Geometry: final body of the model. Coordinates: model frame, mm. Give positions to 0.01 mm unless a question says otherwise; leave off trailing zeros. Write each loop counter-clockwise with the first axis right and the second up, starting at its lowest first coordinate (ties: lowest second). Pieces come first, ordered by that corner, then holes.
Autodesk Inventor part; units mm, degrees
ref_plane "YZ Plane" through (0, 0, 0) normal (1, 0, 0) x (0, 1, 0)
ref_plane "XZ Plane" through (0, 0, 0) normal (0, 1, 0) x (-1, 0, 0)
ref_plane "XY Plane" through (0, 0, 0) normal (0, 0, 1) x (1, 0, 0)
sketch "Sketch3" plane through (0, 0, 0) normal (0, 1, 0) x (-1, 0, 0)
  line L0 (-56.572, -4.0671) -> (-56.572, -54.0671)
  line L1 (-6.572, -54.0671) -> (-6.572, -4.0671)
  line L2 (-6.572, -4.0671) -> (-35.572, -4.0671)
  line L3 (-35.572, -4.0671) -> (-35.572, -8.0671)
  line L4 (-35.572, -8.0671) -> (-27.572, -8.0671)
  line L5 (-27.572, -8.0671) -> (-27.572, -4.0671)
  line L6 (-27.572, -4.0671) -> (-56.572, -4.0671)
  line L7 (-6.572, -29.0671) -> (-22.7851, -29.0671) construction
  line L8 (-6.572, -54.0671) -> (-35.572, -54.0671)
  line L9 (-35.572, -54.0671) -> (-35.572, -50.0671)
  line L10 (-35.572, -50.0671) -> (-27.572, -50.0671)
  line L11 (-27.572, -50.0671) -> (-27.572, -54.0671)
  line L12 (-27.572, -54.0671) -> (-56.572, -54.0671)
  line L13 (-21.572, -4.0671) -> (-21.572, -19.0671) construction
  line L14 (-21.572, -19.0671) -> (-6.572, -19.0671) construction
  line L15 (-56.572, -19.0671) -> (-41.572, -19.0671) construction
  line L16 (-56.572, -39.0671) -> (-41.572, -39.0671) construction
  line L17 (-21.572, -54.0671) -> (-21.572, -39.0671) construction
  line L18 (-21.572, -39.0671) -> (-6.572, -39.0671) construction
  circle A0 centre (-21.572, -19.0671) radius 3
  circle A1 centre (-41.572, -19.0671) radius 3
  circle A2 centre (-41.572, -39.0671) radius 3
  circle A3 centre (-21.572, -39.0671) radius 3
  point P0 (-35.572, -4.0671)
  dimension "d36" = 50
  dimension "d37" = 50
  dimension "d38" = 4
  dimension "d40" = 15
  dimension "d41" = 6
  dimension "d46" = 8
extrude "Extrusion3" add sketch "Sketch3" along normal blind 600 contours L6 L3 L4 L5 L2 L1 L8 L11 L10 L9 L12 L0 | A0 | A1 | A2 | A3
extrude "Extrusion6" cut sketch "Sketch3" along normal blind 30 contours A0 | A1 | A2 | A3
extrude "Extrusion7" cut sketch "Sketch3" against normal blind 30 from surface at 600 contours A0 | A1 | A2 | A3
equation "\"d36\" = inner_leg_width"
equation "\"d37\" = inner_leg_width"
equation "\"d38\" = cabel_shaft_size"
equation "\"d40\" = edge_to_hole"
equation "\"d41\" = hole_diameter"
equation "\"d46\" = 2 * cabel_shaft_size"
equation "\"d12\" = height"
equation "\"d42\" = hole_depth"
equation "\"d44\" = hole_depth"
equation "\"cabel_shaft_size\" = 4"
equation "\"edge_to_hole\" = 15"
equation "\"hole_diameter\" = 6"
equation "\"height\" = 600"
equation "\"inner_leg_width\" = 50"
equation "\"hole_depth\" = 30"
properties part number "1_inner_leg"
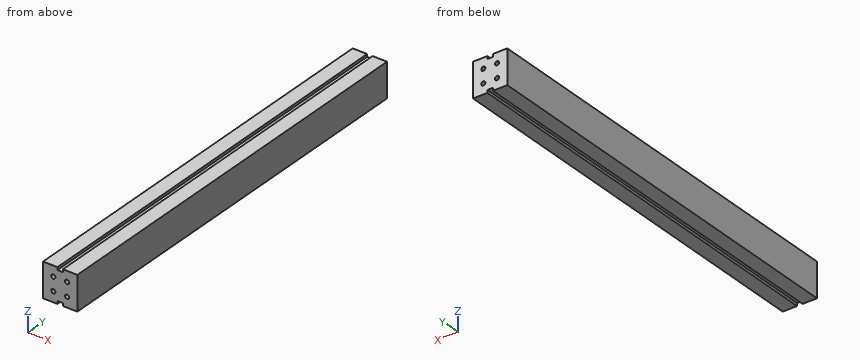
Q1. Section A-A on y = 361. Output: boundary loops of the cut face in (x, z), plus the area to 3 significant figures.
Filled sheet:
outline: (6.57, -54.07) - (27.57, -54.07) - (27.57, -50.07) - (35.57, -50.07) - (35.57, -54.07) - (56.57, -54.07) - (56.57, -4.07) - (35.57, -4.07) - (35.57, -8.07) - (27.57, -8.07) - (27.57, -4.07) - (6.57, -4.07) - close
area: 2,440 mm2
Q2. Ray query, line 1 along Z through (x, y) = (35, 540). Return the intervals inside material, ascending.
Filled sheet:
line 1: z = -50.07 to -8.07
Q3. Pin query (flat end, axial travel): P1, Ø2.5, axis at x = 30, y = 357.5, coming from the -Z side; P2, Ø5.5, axis at x = 21.57, z = -19.07, coming from the +Y side. Return the tip coordinate at first contact, or that it passes through.
Filled sheet:
P1: stops at z = -50.07
P2: stops at y = 570
